from build123d import *

# Parameters (mm, degrees)
SKETCH1_R           = 12.45
SKETCH1_R_2         = 1.7
BOSS_EXTRUDE1_DEPTH = 2.75
SKETCH2_W           = 7.7
SKETCH2_H           = 6.7
BOSS_EXTRUDE2_DEPTH = 3.5
BOSS_EXTRUDE3_START = 1
SKETCH3_R           = 13.5
SKETCH3_R_2         = 1.7
BOSS_EXTRUDE3_DEPTH = 1
CHAMFER1_SIZE       = 1
CHAMFER2_SIZE       = 0.5
CUT_EXTRUDE1_DEPTH  = 2.25
FILLET1_R           = 2.5
CHAMFER3_SIZE       = 1


with BuildPart() as part:
    # Sketch1 → Boss-Extrude1 (new body)
    with BuildSketch(Plane.XY):
        Circle(SKETCH1_R)
        with Locations((-7.36300717, 0)):
            Circle(SKETCH1_R_2, mode=Mode.SUBTRACT)
        with Locations(Location((7.36300717, 0, 0), (0, 0, 180))):
            Circle(SKETCH1_R_2, mode=Mode.SUBTRACT)
    extrude(amount=-BOSS_EXTRUDE1_DEPTH)

    # Sketch2 → Boss-Extrude2 (add)
    with BuildSketch(Plane(origin=(0, 0, -2.75), x_dir=(-1, 0, 0), z_dir=(0, 0, -1))):
        Rectangle(SKETCH2_W, SKETCH2_H)
    extrude(amount=BOSS_EXTRUDE2_DEPTH)

    # Sketch3 → Boss-Extrude3 (add)
    with BuildSketch(Plane.XY.offset(BOSS_EXTRUDE3_START)):
        Circle(SKETCH3_R)
        with Locations((-7.36300717, 0)):
            Circle(SKETCH3_R_2, mode=Mode.SUBTRACT)
        with Locations((7.36300717, 0)):
            Circle(SKETCH3_R_2, mode=Mode.SUBTRACT)
    extrude(amount=-BOSS_EXTRUDE3_DEPTH)

    # Chamfer1
    chamfer1_edges = [part.edges().sort_by_distance(p)[0] for p in [
        (-3.85, 0, -6.25),
        (0, 3.35, -6.25),
        (3.85, 0, -6.25),
        (0, -3.35, -6.25),
        (-12.45, 0, -2.75),
    ]]
    chamfer(chamfer1_edges, length=CHAMFER1_SIZE)

    # Chamfer2
    chamfer2_edges = [part.edges().sort_by_distance(p)[0] for p in [
        (-13.5, 0, 0),
    ]]
    chamfer(chamfer2_edges, length=CHAMFER2_SIZE)

    # Sketch4 → Cut-Extrude1 (cut)
    with BuildSketch(Plane.XY.offset(1)):
        with BuildLine():
            Line((2.54627648, 7.525661596), (2.54627648, -7.525661596))
            ThreePointArc((2.54627648, -7.525661596), (0, -10.071938075), (-2.54627648, -7.525661596))
            Line((-2.54627648, -7.525661596), (-2.54627648, 7.525661596))
            ThreePointArc((-2.54627648, 7.525661596), (0, 10.071938075), (2.54627648, 7.525661596))
        make_face()
    extrude(amount=-CUT_EXTRUDE1_DEPTH, mode=Mode.SUBTRACT)

    # Fillet1
    # the kernel refuses this fillet: 2.5 mm, written as the material it adds along each edge
    with BuildSketch(Plane(origin=(-2.54627648, -7.525661596, -1.25), x_dir=(0, 0, 1), z_dir=(0, 1, 0)), Plane(origin=(2.54627648, 7.525661596, -1.25), x_dir=(0, 0, 1), z_dir=(0, -1, 0))) as fillet1_piece_1:
        with BuildLine():
            CenterArc((2.5, 2.487468593), FILLET1_R, 180, 84.260829523)
            Line((0, 2.487468593), (-0.05, 2.487468593))
            Line((-0.05, 2.487468593), (-0.05, 0))
            Line((-0.05, 0), (0, -0.05))
            ThreePointArc((0, -0.05), (1.125, -0.05), (2.245, -0.049749372))
            Line((2.245, -0.049749372), (2.25, 0))
        make_face()
    extrude(amount=15.051323191)
    with BuildSketch(Plane(origin=(0, 7.525661596, -1.25), x_dir=(-1, 0, 0), z_dir=(0, -1, 0))) as fillet1_piece_2:
        with BuildLine():
            CenterArc((0.058807887, -2.5), FILLET1_R, 5.739170477, 84.260829523)
            Line((0.058807887, 0), (0.058807887, 0.05))
            Line((0.058807887, 0.05), (2.54627648, 0.05))
            Line((2.54627648, 0.05), (2.59627648, 0))
            ThreePointArc((2.59627648, 0), (2.59627648, -1.125), (2.596025852, -2.245))
            Line((2.596025852, -2.245), (2.54627648, -2.25))
        make_face()
    revolve(axis=Axis((0, 7.525661596, -1.25), (0, 0, -1)), revolution_arc=180)
    with BuildSketch(Plane(origin=(0, -7.525661596, -1.25), x_dir=(1, 0, 0), z_dir=(0, 1, 0))) as fillet1_piece_3:
        with BuildLine():
            CenterArc((0.058807887, -2.5), FILLET1_R, 5.739170477, 84.260829523)
            Line((0.058807887, 0), (0.058807887, 0.05))
            Line((0.058807887, 0.05), (2.54627648, 0.05))
            Line((2.54627648, 0.05), (2.59627648, 0))
            ThreePointArc((2.59627648, 0), (2.59627648, -1.125), (2.596025852, -2.245))
            Line((2.596025852, -2.245), (2.54627648, -2.25))
        make_face()
    revolve(axis=Axis((0, -7.525661596, -1.25), (0, 0, -1)), revolution_arc=180)

    # Chamfer3
    # the kernel refuses this chamfer: 1 mm, written as the material it takes off along each edge
    with BuildSketch(Plane(origin=(-7.36300717, 0, 1), x_dir=(1, 0, 0), z_dir=(0, -1, 0))) as chamfer3_piece_1:
        Polygon((1.7 + CHAMFER3_SIZE, 0), (1.7, -CHAMFER3_SIZE), (1.7, 0), align=None)
    revolve(axis=Axis((-7.36300717, 0, 1), (0, 0, 1)), mode=Mode.SUBTRACT)
    with BuildSketch(Plane(origin=(7.36300717, 0, 1), x_dir=(1, 0, 0), z_dir=(0, -1, 0))) as chamfer3_piece_2:
        Polygon((1.7 + CHAMFER3_SIZE, 0), (1.7, -CHAMFER3_SIZE), (1.7, 0), align=None)
    revolve(axis=Axis((7.36300717, 0, 1), (0, 0, 1)), mode=Mode.SUBTRACT)


solid = part.part
The listing builds one solid part. Answer for the finished solid, in the listing's coordinates (mm). A direction names the side the tool comes from. Round coordinates to 2 decimals unless told otherwise and drop trailing zeros. Write each loop counter-clockwise with the first axis right and the second up, starting at its lowest first coordinate (ties: lowest second). Pieces come first, ordered by that corner, then holes. Notation, with made-up numbers: M 67.25,16 L 94.25,16 A15 ccw 94.25,32 Z; hole C 74,20 d3. An arc over 180 degrees is marked long. Write each question's results on one line, items separated by ' | '. Start each with the question number.
Item 1: Find section A-A on y = 0. Give the number of separate pieces and of enclosed holes in the cut face, and give its area (3 significant figures).
Item 2: Which of the six approach directions +Z, -Z, +X, -X, +Y, -Y give full straight-line access (tool end or side, diameter ignored) to faces 4 (the flat face through (-3.85, 0, -4)), 5 (the cylindrical face through (-9.18, 8.41, -0.86)), 6 (the cylindrical face through (1.72, 0.11, -0.62)), 7 (the flat face through (0, -3.35, -4)), 8 (the flat face through (3.85, 0, -4))?
Item 3: Straight lines are drawn through the part: probe 1 along X at (y, z) = (-0.5, -0.75); probe 2 along X at (y, z) = (0.5, -0.5); probe 3 along Z at (x, y) = (-6, 5.25). For each, find the intervals that lie inside material, in ascending order.
Item 4: Given pin 1 Ø4 at (y, z) = (-5, -4.5) entering from +X; pin 2 Ø1.2 at (x, z) = (0.5, -4) entering from -Y; pin 3 Ø1.5 at (y, z) = (-6.5, -2) entering from +X, each flat-ended and moving along its own axis, determine where each tip first touches the part or whether it passes through.
Item 5: The mould has two halves that part along Y. Classify faces 1 (the flat face through (5, 0, -2.75)), 2 (the cylindrical face through (-9.06, 0.07, -1.36)), 3 (the flat face through (0, 3.35, -4)): +Y half, -Y half, draft (parallel to the pull), parting line (faces both ways), or undercut.
Item 6: Find section B-B on z = -3.5. Write down the section's boundary in (x, y).
Answer block:
1) separate pieces: 3 | enclosed holes: 0 | area: 83.8 mm²
2) face 4: -Z, -X, +Y, -Y | face 5: -Z | face 6: +Z | face 7: -Z, +X, -X, -Y | face 8: -Z, +X, +Y, -Y
3) probe 1: x = -12.44 to -8.99, -5.74 to -1.56, 1.56 to 5.74, 8.99 to 12.44 | probe 2: x = -12.44 to -8.99, -5.74 to -1.84, 1.84 to 5.74, 8.99 to 12.44 | probe 3: z = -2.75 to 1
4) pin 1: stops at x = 10.75 | pin 2: stops at y = -3.35 | pin 3: stops at x = 11.02
5) face 1: draft | face 2: undercut | face 3: +Y half
6) outline: M -3.85,-3.35 L 3.85,-3.35 L 3.85,3.35 L -3.85,3.35 Z
